```python
from build123d import *

# Parameters (mm, degrees)
SKETCH1_R               = 1.5
BOSS_EXTRUDE1_DEPTH     = 6
BOSS_EXTRUDE2_DEPTH     = 4
CUT_EXTRUDE1_DEPTH      = 5
CUT_EXTRUDE1_DEPTH_BACK = 7
SKETCH3_R               = 2
BOSS_EXTRUDE3_DEPTH     = 3
FILLET1_R               = 2
SKETCH4_R               = 1.5
BOSS_EXTRUDE4_DEPTH     = 2


with BuildPart() as part:
    # Sketch1 → Boss-Extrude1 (new body)
    with BuildSketch(Plane.XY):
        with BuildLine():
            Line((1, 0), (139, 0))
            ThreePointArc((139, 0), (139.707106781, 0.292893219), (140, 1))
            Line((140, 1), (140, 55))
            ThreePointArc((140, 55), (139.707106781, 55.707106781), (139, 56))
            Line((139, 56), (1, 56))
            ThreePointArc((1, 56), (0.292893219, 55.707106781), (0, 55))
            Line((0, 55), (0, 1))
            ThreePointArc((0, 1), (0.292893219, 0.292893219), (1, 0))
        make_face()
        with Locations((5.5, 51.5)):
            Circle(SKETCH1_R, mode=Mode.SUBTRACT)
        with Locations((5.5, 4.5)):
            Circle(SKETCH1_R, mode=Mode.SUBTRACT)
        with Locations((134.5, 4.5)):
            Circle(SKETCH1_R, mode=Mode.SUBTRACT)
        with Locations((134.5, 51.5)):
            Circle(SKETCH1_R, mode=Mode.SUBTRACT)
    extrude(amount=-BOSS_EXTRUDE1_DEPTH)

    # Sketch1<3> → Boss-Extrude2 (add)
    with BuildSketch(Plane.XY):
        with BuildLine():
            ThreePointArc((0, 1), (0.292893219, 0.292893219), (1, 0))
            Line((1, 0), (139, 0))
            ThreePointArc((139, 0), (139.707106781, 0.292893219), (140, 1))
            Line((140, 1), (140, 55))
            ThreePointArc((140, 55), (139.707106781, 55.707106781), (139, 56))
            Line((139, 56), (1, 56))
            ThreePointArc((1, 56), (0.292893219, 55.707106781), (0, 55))
            Line((0, 55), (0, 1))
        make_face()
        with BuildLine():
            ThreePointArc((2, 53.5), (2.292893219, 54.207106781), (3, 54.5))
            Line((3, 54.5), (137, 54.5))
            ThreePointArc((137, 54.5), (137.707106781, 54.207106781), (138, 53.5))
            Line((138, 53.5), (138, 2.5))
            ThreePointArc((138, 2.5), (137.707106781, 1.792893219), (137, 1.5))
            Line((137, 1.5), (3, 1.5))
            ThreePointArc((3, 1.5), (2.292893219, 1.792893219), (2, 2.5))
            Line((2, 2.5), (2, 53.5))
        make_face(mode=Mode.SUBTRACT)
    extrude(amount=BOSS_EXTRUDE2_DEPTH)

    # Sketch2 → Cut-Extrude1 (cut, two sides)
    with BuildSketch(Plane.XY) as cut_extrude1_sk:
        with BuildLine():
            Line((11, 49.5), (129, 49.5))
            ThreePointArc((129, 49.5), (131.828427125, 48.328427125), (133, 45.5))
            Line((133, 45.5), (133, 10.5))
            ThreePointArc((133, 10.5), (131.828427125, 7.671572875), (129, 6.5))
            Line((129, 6.5), (11, 6.5))
            ThreePointArc((11, 6.5), (8.171572875, 7.671572875), (7, 10.5))
            Line((7, 10.5), (7, 45.5))
            ThreePointArc((7, 45.5), (8.171572875, 48.328427125), (11, 49.5))
        make_face()
    extrude(amount=CUT_EXTRUDE1_DEPTH, mode=Mode.SUBTRACT)
    extrude(cut_extrude1_sk.sketch, amount=-CUT_EXTRUDE1_DEPTH_BACK, mode=Mode.SUBTRACT)

    # Sketch3 → Boss-Extrude3 (add)
    with BuildSketch(Plane(origin=(0, 0, -6), x_dir=(-1, 0, 0), z_dir=(0, 0, -1))):
        with BuildLine():
            Line((-6.5, 0), (-6.5, -5))
            ThreePointArc((-6.5, -5), (-7.378679656, -7.121320344), (-9.5, -8))
            Line((-9.5, -8), (-10.5, -8))
            ThreePointArc((-10.5, -8), (-12.621320344, -7.121320344), (-13.5, -5))
            Line((-13.5, -5), (-13.5, 0))
            Line((-13.5, 0), (-6.5, 0))
        make_face()
        with Locations((-10, -4)):
            Circle(SKETCH3_R, mode=Mode.SUBTRACT)
        with BuildLine():
            Line((-6.5, 56), (-13.5, 56))
            Line((-13.5, 56), (-13.5, 61))
            ThreePointArc((-13.5, 61), (-12.621320344, 63.121320344), (-10.5, 64))
            Line((-10.5, 64), (-9.5, 64))
            ThreePointArc((-9.5, 64), (-7.378679656, 63.121320344), (-6.5, 61))
            Line((-6.5, 61), (-6.5, 56))
        make_face()
        with Locations((-10, 60)):
            Circle(SKETCH3_R, mode=Mode.SUBTRACT)
        with BuildLine():
            Line((-126.5, 56), (-126.5, 61))
            ThreePointArc((-126.5, 61), (-127.378679656, 63.121320344), (-129.5, 64))
            Line((-129.5, 64), (-130.5, 64))
            ThreePointArc((-130.5, 64), (-132.621320344, 63.121320344), (-133.5, 61))
            Line((-133.5, 61), (-133.5, 56))
            Line((-133.5, 56), (-126.5, 56))
        make_face()
        with Locations((-130, 60)):
            Circle(SKETCH3_R, mode=Mode.SUBTRACT)
        with BuildLine():
            Line((-133.5, 0), (-133.5, -5))
            ThreePointArc((-133.5, -5), (-132.621320344, -7.121320344), (-130.5, -8))
            Line((-130.5, -8), (-129.5, -8))
            ThreePointArc((-129.5, -8), (-127.378679656, -7.121320344), (-126.5, -5))
            Line((-126.5, -5), (-126.5, 0))
            Line((-126.5, 0), (-133.5, 0))
        make_face()
        with Locations((-130, -4)):
            Circle(SKETCH3_R, mode=Mode.SUBTRACT)
    extrude(amount=-BOSS_EXTRUDE3_DEPTH)

    # Fillet1
    fillet1_edges = [part.edges().sort_by_distance(p)[0] for p in [
        (13.5, 0, -4.5),
        (6.5, 0, -4.5),
        (6.5, 56, -4.5),
        (13.5, 56, -4.5),
        (126.5, 56, -4.5),
        (133.5, 56, -4.5),
        (133.5, 0, -4.5),
        (126.5, 0, -4.5),
    ]]
    fillet(fillet1_edges, radius=FILLET1_R)

    # Sketch4 → Boss-Extrude4 (add)
    with BuildSketch(Plane.XY):
        with BuildLine():
            Line((8.5, 51.5), (8.5, 54.880942349))
            Line((8.5, 54.880942349), (6, 54.880942349))
            Line((6, 54.880942349), (1.461490173, 54.880942349))
            Line((1.461490173, 54.880942349), (1.461490173, 48.5))
            Line((1.461490173, 48.5), (5.5, 48.5))
            ThreePointArc((5.5, 48.5), (7.621320344, 49.378679656), (8.5, 51.5))
        make_face()
        with Locations((5.5, 51.5)):
            Circle(SKETCH4_R, mode=Mode.SUBTRACT)
        with BuildLine():
            Line((134, 54.880942349), (131.5, 54.880942349))
            Line((131.5, 54.880942349), (131.5, 51.5))
            ThreePointArc((131.5, 51.5), (132.378679656, 49.378679656), (134.5, 48.5))
            Line((134.5, 48.5), (138.538509827, 48.5))
            Line((138.538509827, 48.5), (138.538509827, 54.880942349))
            Line((138.538509827, 54.880942349), (134, 54.880942349))
        make_face()
        with Locations((134.5, 51.5)):
            Circle(SKETCH4_R, mode=Mode.SUBTRACT)
        with BuildLine():
            Line((131.5, 4.5), (131.5, 1.119057651))
            Line((131.5, 1.119057651), (134, 1.119057651))
            Line((134, 1.119057651), (138.538509827, 1.119057651))
            Line((138.538509827, 1.119057651), (138.538509827, 7.5))
            Line((138.538509827, 7.5), (134.5, 7.5))
            ThreePointArc((134.5, 7.5), (132.378679656, 6.621320344), (131.5, 4.5))
        make_face()
        with Locations((134.5, 4.5)):
            Circle(SKETCH4_R, mode=Mode.SUBTRACT)
        with BuildLine():
            Line((6, 1.119057651), (8.5, 1.119057651))
            Line((8.5, 1.119057651), (8.5, 4.5))
            ThreePointArc((8.5, 4.5), (7.621320344, 6.621320344), (5.5, 7.5))
            Line((5.5, 7.5), (1.461490173, 7.5))
            Line((1.461490173, 7.5), (1.461490173, 1.119057651))
            Line((1.461490173, 1.119057651), (6, 1.119057651))
        make_face()
        with Locations((5.5, 4.5)):
            Circle(SKETCH4_R, mode=Mode.SUBTRACT)
    extrude(amount=BOSS_EXTRUDE4_DEPTH)


solid = part.part
```
Here's how the part is built. I have some questions about the finished solid (model axes, mm). A direction names the side the tool comes from. Coordinates: 2 decimals unless noted, no trailing zeros. Order: outer loops, then holes, each group sorted by start corner. A loop starts at its lowest first (then second) coordinate and runs counter-clockwise, first axis right, second up.
Item 1: I'm going to push flat-ended pins straight in: pin 1 Ø3 at (x, y) = (10, 60) entering from +Z; pin 2 Ø0.9 at (y, z) = (-4, -4.5) entering from -X; pin 3 Ø3 at (x, z) = (92, 2) entering from -Y; pin 4 Ø1.6 at (x, z) = (3.5, 1.5) entering from +Y. Where does each tip first touch, or does it pass through?
Response values:
pin 1: passes through
pin 2: stops at x = 6.5
pin 3: stops at y = 0
pin 4: stops at y = 56
Item 2: If we section it at B-B, the plane y = 43.5: List the corners of the cut face in (x, z) for me.
Response values:
outline: (0, -6) - (7, -6) - (7, 0) - (2, 0) - (2, 4) - (0, 4) - close; (133, -6) - (140, -6) - (140, 4) - (138, 4) - (138, 0) - (133, 0) - close
Item 3: I need wall thicknesses on probe 1 along Y at (x, z) = (5.5, -2.5); probe 2 along Y at (x, z) = (53, -0.5); probe 3 along Y at (x, z) = (99.5, 1). Which ranges of each line are inside material? Lowest first, please.
Response values:
probe 1: y = 0 to 3, 6 to 50, 53 to 56
probe 2: y = 0 to 6.5, 49.5 to 56
probe 3: y = 0 to 1.5, 54.5 to 56
Item 4: Thinking about a two-plate mould opening in X: for faces 1 (the face through (6.5, -3, -5)), 2 (the face through (71, 6.5, -3)), 3 (the face through (75, 50, -6)), which applies, pulls with the +X half, pulls with the -X half, needs draft (parallel to the pull), parting line crosses it, or undercut?
Response values:
face 1: pulls with the -X half
face 2: undercut
face 3: needs draft
Item 5: If we section it at A-A, the plane x = 97.5: List the corners of the cut face in (y, z) for me, then the cut area to 3 significant figures.
Response values:
outline: (0, -6) - (6.5, -6) - (6.5, 0) - (1.5, 0) - (1.5, 4) - (0, 4) - close; (49.5, -6) - (56, -6) - (56, 4) - (54.5, 4) - (54.5, 0) - (49.5, 0) - close
area: 90.0 mm2
Item 6: If we section it at C-C, the plane z = -1.5: List the corners of the cut face in (x, y) for me.
Response values:
outline: (0, 1) arc R1 ccw to (1, 0) - (139, 0) arc R1 ccw to (140, 1) - (140, 55) arc R1 ccw to (139, 56) - (1, 56) arc R1 ccw to (0, 55) - close; hole circle Ø3 at (5.5, 4.5); hole circle Ø3 at (5.5, 51.5); hole (7, 10.5) arc R4 ccw to (11, 6.5) - (129, 6.5) arc R4 ccw to (133, 10.5) - (133, 45.5) arc R4 ccw to (129, 49.5) - (11, 49.5) arc R4 ccw to (7, 45.5) - close; hole circle Ø3 at (134.5, 4.5); hole circle Ø3 at (134.5, 51.5)
Item 7: Which directions (+Z, -Z, +X, -X, +Y, -Y) give clear straight access to the entire face, cutting with the end or side of a thin tool? Please do faces 4 (the face through (7, 28, -3)), 5 (the face through (129, -2, -3)), 6 (the face through (71, 1.5, 2)), 7 (the face through (71, 56, -1)).
Response values:
face 4: +Z, -Z
face 5: +Z, +X, -X, -Y
face 6: +Z
face 7: +Z, +Y
